from build123d import *

# Parameters (mm, degrees)
F4_SCALE = 1.3


# Not quite as in the source:
# - ends of sketch curves that miss each other by under 0.0002 mm in the source are joined
# - a feature of the source that left no trace in its solid (it failed there, or was rolled back) is left out


with BuildPart() as f1:
    # F0 (on Right) → F1 (revolve)
    with BuildSketch(Plane.YZ):
        with BuildLine():
            Line((-10, 10), (-10, 0))
            Line((-10, 0), (10, 0))
            Line((10, 0), (10, 10))
            Line((10, 10), (7.5, 10))
            add(Edge.make_bspline(
                [(7.5, 10), (6.3198292539, 10.0170777093), (6.0755360942, 16.2900794914), (8.71740503, 20.4397404153), (14.1975799439, 22.3834382863), (15.4026740679, 23.9286791718), (15.4000005056, 25)],
                knots=[0, 0, 0, 0, 0.2720899799, 0.5413764913, 0.8105016424, 1, 1, 1, 1], degree=3))
            Line((15.4000005056, 25), (15.5000005056, 25))
            Line((15.5000005056, 25), (15.5000005056, 30))
            Line((15.5000005056, 30), (15.0000005056, 30))
            add(Edge.make_bspline(
                [(15.0000005056, 30), (15.0842336639, 34.1735254493), (15.4036855603, 41.6818231934), (14.026949329, 49.0386767347), (12.0611475076, 50.0140784293), (10.0000005056, 50)],
                knots=[0, 0, 0, 0, 0.4362070764, 0.7559396549, 1, 1, 1, 1], degree=3))
            Line((10.0000005056, 50), (5.056e-07, 50))
            Line((5.056e-07, 50), (-10.0000005056, 50))
            add(Edge.make_bspline(
                [(-15.0000005056, 30), (-15.0842336639, 34.1735254493), (-15.4036855603, 41.6818231934), (-14.026949329, 49.0386767347), (-12.0611475076, 50.0140784293), (-10.0000005056, 50)],
                knots=[0, 0, 0, 0, 0.4362070764, 0.7559396549, 1, 1, 1, 1], degree=3))
            Line((-15.0000005056, 30), (-15.5000005056, 30))
            Line((-15.5000005056, 30), (-15.5000005056, 25))
            Line((-15.5000005056, 25), (-15.4000005056, 25))
            add(Edge.make_bspline(
                [(-7.5, 10), (-6.3198292539, 10.0170777093), (-6.0755360942, 16.2900794914), (-8.71740503, 20.4397404153), (-14.1975799439, 22.3834382863), (-15.4026740679, 23.9286791718), (-15.4000005056, 25)],
                knots=[0, 0, 0, 0, 0.2720899799, 0.5413764913, 0.8105016424, 1, 1, 1, 1], degree=3))
            Line((-7.5, 10), (-10, 10))
        make_face()
    revolve(axis=Axis((0, 0, 0), (0, 1, 0)))


with BuildPart() as f1_1:
    # F4: moved
    add(f1.part.scale(F4_SCALE))


solid = f1_1.part
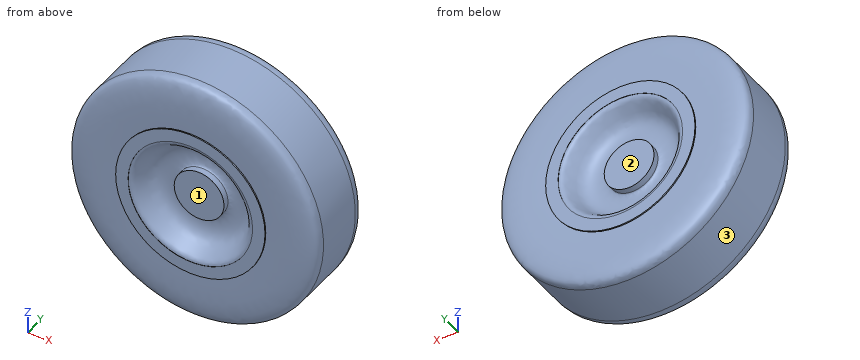
CAD build for the part. Positions are in the model's coordinates, mm. Face numbers are marked on the shaded views. Give positions to 0.01 mm unless a question says otherwise; leave off trailing zeros. Loops run counter-clockwise (first coordinate to the right, second up) from the corner with the lowest first, then second, coordinate; pieces in that order, holes last. Notation, with made-up numbers: M 48,80 L 88,80 A19 ccw 88,107 Z; hole C 75.25,-13 d11. An arc over 180 degrees is marked long. Answer in a Markdown table with one row per item. Add a question column.
Item 1: Drop flat-ended pins along their axis: P1, Ø5, axis at x = -11, y = -11.5, coming from the +Z side; P2, Ø3, axis at y = -9.5, z = -34.5, coming from the -X side; P3, Ø1, axis at x = -10.5, y = -11.5, coming from the +Z side. Give the stop position or say it passes through.
Item 2: Band-saw the part on A-A on y = 4.5. Give the cut face in (x, z).
Item 3: Mould opens along Z. For the marked faces 1, 2 and 3 say: +Z half, -Z half, draft (parallel to the pull), parting line (faces both ways), or undercut.
Item 4: Probe probe 1 along X at (y, z) = (-20.1, 0); probe 2 along Z at (x, y) = (22.5, -11.5); probe 3 along Y at (x, z) = (44, -26). List the from-to ranges inside material, lowest first.
Reply:
| question | item | result |
|---|---|---|
| 1 | P1 | stops at z = 64.44 |
| 1 | P2 | stops at x = -56 |
| 1 | P3 | stops at z = 64.23 |
| 2 | outline | C 0,0 d130 |
| 3 | face 1 | undercut |
| 3 | face 2 | undercut |
| 3 | face 3 | parting line |
| 4 | probe 1 | x = -39 to -32.5, 32.5 to 39 |
| 4 | probe 2 | z = -60.98 to -12.4, 12.4 to 60.98 |
| 4 | probe 3 | y = -19.66 to 19.66 |
